Source: three-view drawing plus pictorial views. Frame: mm from the lowest corner of the part. A direction names the side the tool comes from. Coordinates: 2 decimals unless noted, no trailing zeros. Write each loop counter-clockwise with the first axis right and the second up, starting at its lowest first coordinate (ties: lowest second). Pieces come first, ordered by that corner, then holes. Notation, with made-up numbers: (-26, -37) - (25, -37) arc R12 ccw to (25, -29) - close; hole circle Ø6 at (65, 89). An arc over 180 degrees is marked (long way). Put each result on its own line as item: value.
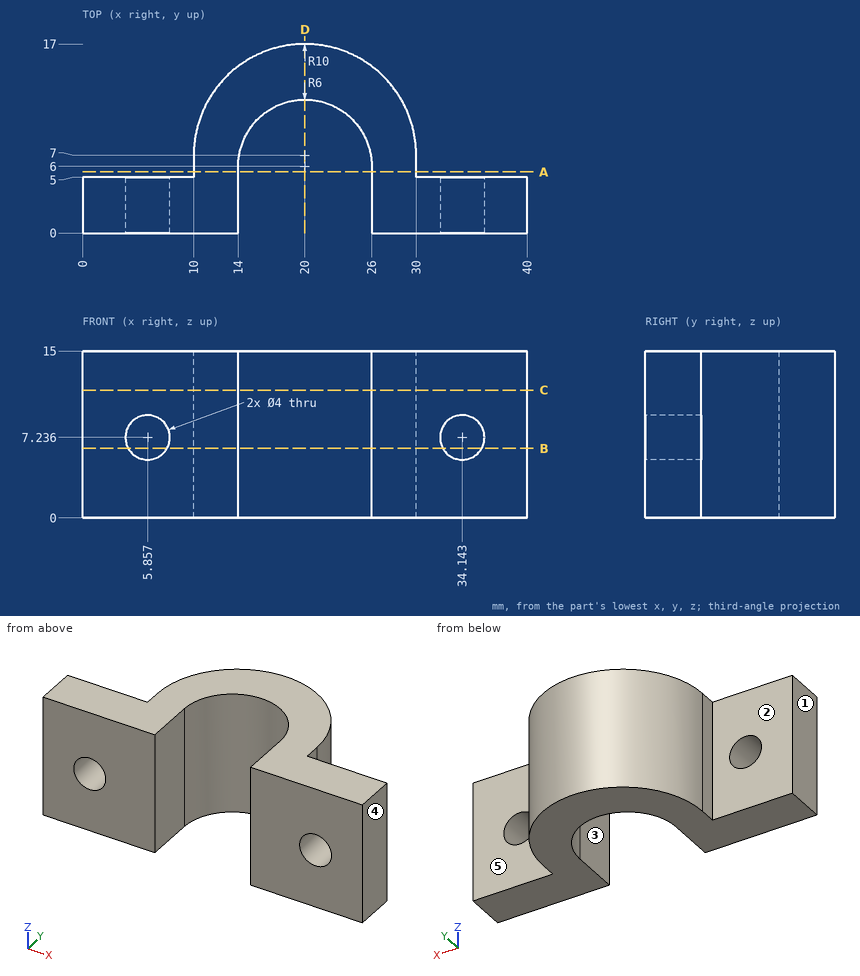
1. Set-up query: the marked faces 1, 2, 3, 4 and 5. Return all of +Z, -Z, +X, -X, +Y, -Y with unobstructed straight access to the full face (end or side cutting, diameter ignored); none if empty.
Answer below:
face 1: +Z, -Z, -X, +Y, -Y
face 2: +Z, -Z, -X, +Y
face 3: +Z, -Z, -Y
face 4: +Z, -Z, +X, +Y, -Y
face 5: +Z, -Z, +X, +Y
2. Ray query, probe 1 along X at (y, z) = (4, 12.25); probe 2 along Y at (x, z) = (2.5, 13.25); probe 3 along X at (y, z) = (15, 2). Return the intervals inside material, ascending. Write a range as from..to.
Answer below:
probe 1: x = 0..14, 26..40
probe 2: y = 0..5
probe 3: x = 14..26
3. Section query A-A (y = 5.5). Return loops of the section in (x, z), then the cut area to 3 significant figures.
Answer below:
outline: (10, 0) - (14, 0) - (14, 15) - (10, 15) - close; (26, 0) - (30, 0) - (30, 15) - (26, 15) - close
area: 120 mm²
4. Pin query (flat end, axial travel): pin 1 Ø3 at (x, y) = (16, 2) entering from +Z; pin 2 Ø8 at (x, z) = (5, 7.5) entering from +Y; pin 3 Ø2 at (y, z) = (8.5, 8.5) entering from -X; pin 4 Ø8 at (y, z) = (14, 4) entering from +X. Return the tip coordinate at first contact, or that it passes through.
Answer below:
pin 1: passes through
pin 2: stops at y = 5
pin 3: stops at x = 10.01
pin 4: stops at x = 29.54
5. Section query C-C (z = 11.5). Return loops of the section in (x, y).
Answer below:
outline: (0, 0) - (14, 0) - (14, 6) arc R6 cw to (26, 6) - (26, 0) - (40, 0) - (40, 5) - (30, 5) - (30, 7) arc R10 ccw to (10, 7) - (10, 5) - (0, 5) - close
6. Section query D-D (x = 20). Return loops of the section in (y, z).
Answer below:
outline: (12, 0) - (17, 0) - (17, 15) - (12, 15) - close
7. Section query B-B (z = 6.25). Return loops of the section in (x, y).
Answer below:
outline: (0, 0) - (4.12, 0) - (4.12, 5) - (0, 5) - close; (7.6, 0) - (14, 0) - (14, 6) arc R6 cw to (26, 6) - (26, 0) - (32.4, 0) - (32.4, 5) - (30, 5) - (30, 7) arc R10 ccw to (10, 7) - (10, 5) - (7.6, 5) - close; (35.88, 0) - (40, 0) - (40, 5) - (35.88, 5) - close
